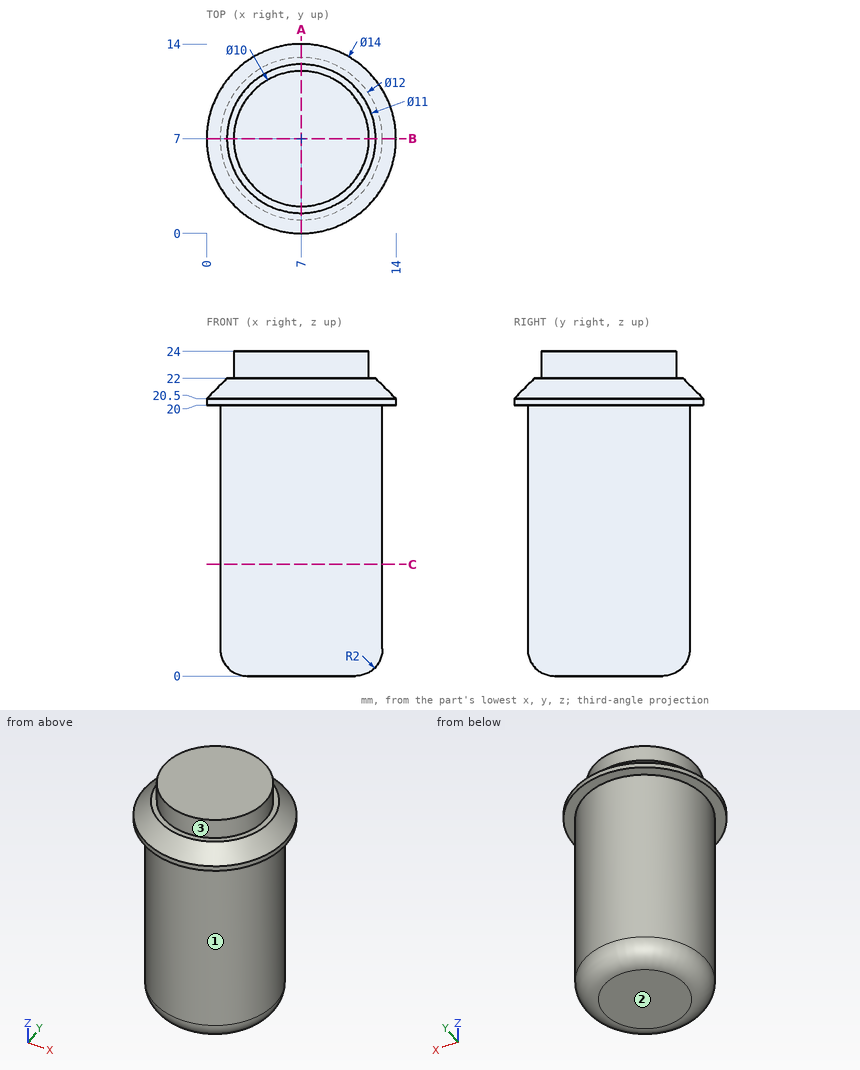
The drawing under review shows one solid part. Ordinate dimensions are in mm from its lowest x, y, z. A direction names the side the tool comes from. Coordinates: 2 decimals unless noted, no trailing zeros. Order: outer loops, then holes, each group sorted by start corner. A loop starts at its lowest first (then second) coordinate and runs counter-clockwise, first axis right, second up. Notation, with made-up numbers: (14, -32.5) -> (67, -32.5) arc R23 cw to (67, -8.5) -> close; hole circle Ø9 at (29, 86.25). An arc over 180 degrees is marked (long way). Answer in a Markdown table with one row per item. Add a question column.
Item 1: To check wall thickness, follow probe 1 along Y at (x, z) = (7, 5.5); probe 2 along Z at (x, y) = (6, 11); probe 3 along X at (y, z) = (7.75, 21.5). State the ranges of each line that lie inside material, in increasing order.
Item 2: We need section A-A on x = 7. Write out the cut boundary in (y, z), plus the area to 3 significant figures.
Item 3: Machinability: for the marked faces 1, 2 and 3, which of the approach directions +Z, -Z, +X, -X, +Y, -Y give a long, thin tool a straight path to every point of the face, cutting with its end or side? Answer none if there is none.
Item 4: Clearance check with flat-ended pins moving along their axes: pin 1 (3 mm diameter, centred on x = 6, y = 9, fed in from -Z); pin 2 (6 mm diameter, centred on x = 2.5, z = 5.5, fed in from +Y); pin 3 (8 mm diameter, centred on x = 7, z = 11, fed in from -Y); pin 4 (2 mm diameter, centred on y = 4.5, z = 21, fed in from +X). State where each tip first meets the part, or that it passes through.
Item 5: We need section C-C on z = 8.25. Write out the cut boundary in (x, y).
Final values:
| question | item | result |
|---|---|---|
| 1 | probe 1 | y = 1 to 13 |
| 1 | probe 2 | z = 0 to 24 |
| 1 | probe 3 | x = 1.05 to 12.95 |
| 2 | outline | (0, 20) -> (1, 20) -> (1, 2) arc R2 ccw to (3, 0) -> (11, 0) arc R2 ccw to (13, 2) -> (13, 20) -> (14, 20) -> (14, 20.5) -> (12.5, 22) -> (12, 22) -> (12, 24) -> (2, 24) -> (2, 22) -> (1.5, 22) -> (0, 20.5) -> close |
| 2 | area | 284 mm2 |
| 3 | face 1 | -Z |
| 3 | face 2 | -Z, +X, -X, +Y, -Y |
| 3 | face 3 | +Z |
| 4 | pin 1 | stops at z = 0 |
| 4 | pin 2 | stops at y = 12.81 |
| 4 | pin 3 | stops at y = 1 |
| 4 | pin 4 | stops at x = 13.81 |
| 5 | outline | circle Ø12 at (7, 7) |
